```python
from build123d import *

# Parameters (mm, degrees)
F0_W     = 90
F0_H     = 10
F1_DEPTH = 10
F2_T     = -2.5
F3_W     = 7.5
F3_H     = 3
F4_DEPTH = 2.5
F5_W     = 3
F5_H     = 10
F6_DEPTH = 7.5
F7_W     = 3
F7_H     = 3
F8_DEPTH = 3


with BuildPart() as f1:
    # F0 (on Top) → F1 (new body)
    with BuildSketch(Plane.XY):
        with Locations((14.77346, -2.340722)):
            Rectangle(F0_W, F0_H)
    extrude(amount=F1_DEPTH)

    # F2
    f2_openings = [f1.faces().sort_by_distance(p)[0] for p in [
        (59.77346, -2.340722, 5),
        (-30.22654, -2.340722, 5),
    ]]
    offset(amount=F2_T, openings=f2_openings)

    # F3 (on face) → F4 (cut, through all)
    with BuildSketch(Plane.XY.offset(10)):
        with Locations((39.516613, -2.340722)):
            Rectangle(F3_W, F3_H)
    extrude(amount=-F4_DEPTH, mode=Mode.SUBTRACT)

    # F5 (on face) → F6 (join)
    with BuildSketch(Plane.XY.offset(10)):
        with Locations((25.61603, -2.340722)):
            Rectangle(F5_W, F5_H)
    extrude(amount=F6_DEPTH)

    # F7 (on face) → F8 (cut)
    with BuildSketch(Plane.XY.offset(17.5)):
        with Locations((25.61603, -2.340722)):
            Rectangle(F7_W, F7_H)
    extrude(amount=-F8_DEPTH, mode=Mode.SUBTRACT)


solid = f1.part
```
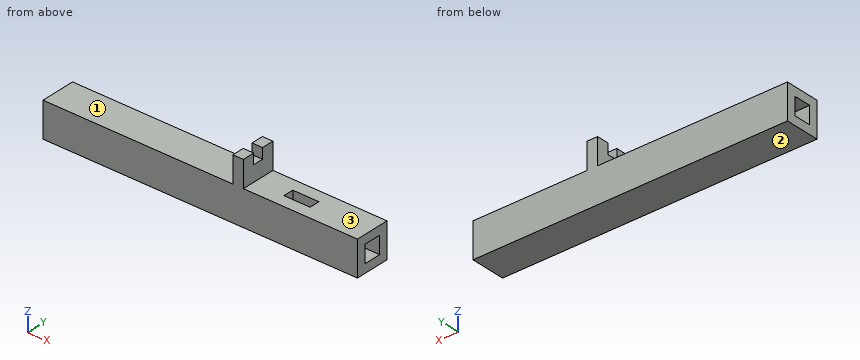
Input: part model. Units: mm. Frame: model coordinates. Face numbers are marked on the shaded views. A direction names the side the tool comes from. Give positions to 0.01 mm unless a question says otherwise; leave off trailing zeros. Write each loop counter-clockwise with the first axis right and the second up, starting at its lowest first coordinate (ties: lowest second). Pieces come first, ordered by that corner, then holes. Notation, with made-up numbers: (46.25, 76) - (105.25, 76) arc R33 cw to (105.25, 114) - close; hole circle Ø8 at (75.5, 55). An arc over 180 degrees is marked (long way). Write item = value, one per line. Start each with the question number.
1. Section query D-D, the plane y = -6.5. Output: boundary loops of the cut face in (x, z).
2. Access query for the marked faces 1, 2 and 3. Directions: +Z, -Z, +X, -X, +Y, -Y. A direction counts if a zero-diameter tool reaches every point of the face in a straight line with its end or side. Return the directions, or none.
3. Section query A-A, the plane y = -2.5. Output: boundary loops of the cut face in (x, z), then the cut area to 3 significant figures.
4. Section query C-C, the plane z = 4.5. Output: boundary loops of the cut face in (x, y), then the cut area to 3 significant figures.
5. Section query B-B, the plane x = 10. Output: boundary loops of the cut face in (y, z), then the cut area to 3 significant figures.
6. Ray query, L1, parallel to Z at x = -14.5, y = -4.25; L2, parallel to Z at x = 24.5, y = -2; L3, parallel to Y at x = 49, z = 6.5. Return the intervals inside material, ascending.
7. First-contact query: pin 1 Ø2.5 at (x, y) = (-5.5, -1) entering from +Z. Flat tip, straight axial feed; report the tip coordinate or a pass-through.
Check sheet entries:
q1.outline = (-30.23, 0) - (59.77, 0) - (59.77, 10) - (27.12, 10) - (27.12, 17.5) - (24.12, 17.5) - (24.12, 10) - (-30.23, 10) - close
q2.face_1 = +Z, -X, +Y, -Y
q2.face_2 = -Z, +X, -X, +Y, -Y
q2.face_3 = +Z, +X, +Y, -Y
q3.outline = (-30.23, 0) - (59.77, 0) - (59.77, 2.5) - (-30.23, 2.5) - close; (-30.23, 7.5) - (35.77, 7.5) - (35.77, 10) - (27.12, 10) - (27.12, 14.5) - (24.12, 14.5) - (24.12, 10) - (-30.23, 10) - close; (43.27, 7.5) - (59.77, 7.5) - (59.77, 10) - (43.27, 10) - close
q3.area = 445 mm2
q4.outline = (-30.23, -7.34) - (59.77, -7.34) - (59.77, -4.84) - (-30.23, -4.84) - close; (-30.23, 0.16) - (59.77, 0.16) - (59.77, 2.66) - (-30.23, 2.66) - close
q4.area = 450 mm2
q5.outline = (-7.34, 0) - (2.66, 0) - (2.66, 10) - (-7.34, 10) - close; hole (-4.84, 2.5) - (0.16, 2.5) - (0.16, 7.5) - (-4.84, 7.5) - close
q5.area = 75.0 mm2
q6.L1 = 0 to 2.5, 7.5 to 10
q6.L2 = 0 to 2.5, 7.5 to 14.5
q6.L3 = -7.34 to -4.84, 0.16 to 2.66
q7.pin_1 = 10
